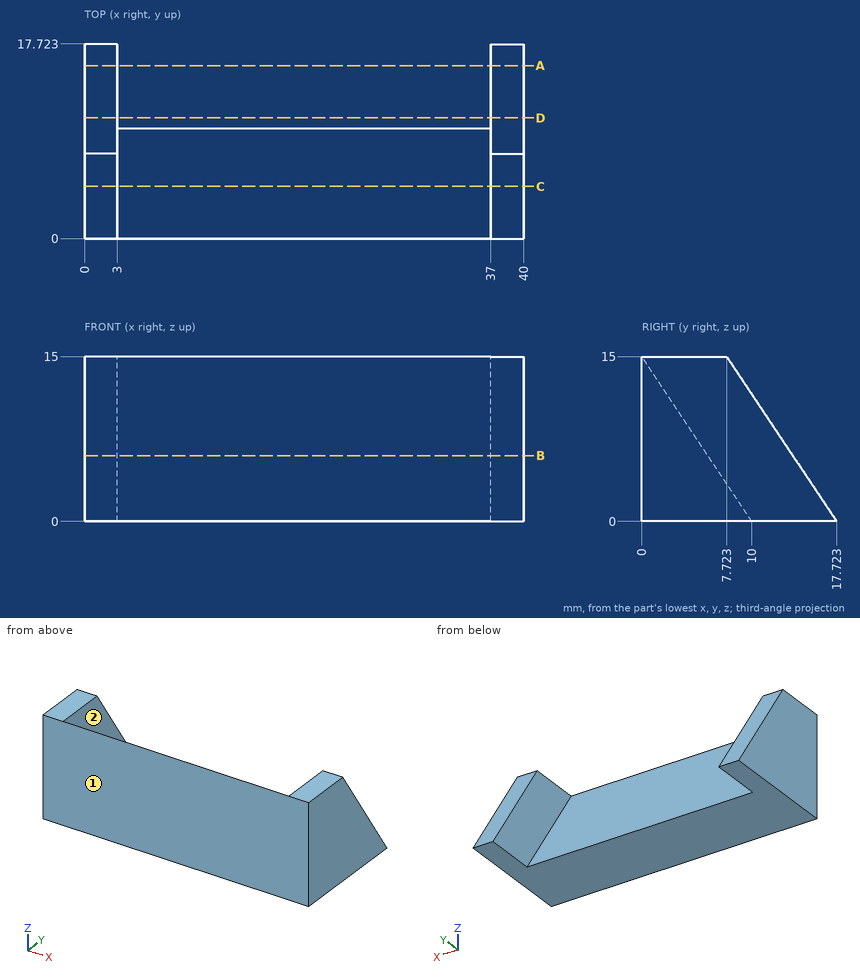
For this review, use the dimensioned drawing (mm, ordinates from the lowest corner) and the shaded views. A direction names the side the tool comes from. Coordinates: 2 decimals unless noted, no trailing zeros. Loops run counter-clockwise (first coordinate to the right, second up) from the corner with the lowest first, then second, coordinate; pieces in that order, holes last. Notation, with made-up numbers: (44.25, -34.5) -> (59.25, -34.5) arc R17 cw to (59.25, -14.5) -> close; hole circle Ø5 at (-37, -6). An arc over 180 degrees is marked (long way). Use a Markdown table: item, result. Add a question column.
1. Add section D-D on y = 11. Write out the cut boundary in (x, z).
2. Clearance check with flat-ended pins moving along their axes: pin 1 Ø8 at (y, z) = (13, 4.5) entering from -X; pin 2 Ø5 at (x, y) = (6, 9.5) entering from +Z; pin 3 Ø6 at (x, z) = (27.5, 6) entering from +Y; pin 4 Ø5 at (y, z) = (13.5, 13) entering from -X. State where each tip first meets the part, or that it passes through.
3. Add section B-B on z = 6. Write out the cut boundary in (x, y).
4. To check wall thickness, follow line 1 (X direction, y = 11, z = 3.5); line 2 (Z direction, x = 21.5, y = 8); line 3 (Z direction, x = 14, y = 3.25) (1 decimal). State the ranges of each line that lie inside material, in increasing order.
5. Machinability: for the marked faces 1 and 2, which of the approach directions +Z, -Z, +X, -X, +Y, -Y give a long, thin tool a straight path to every point of the face, cutting with its end or side? Answer none if there is none.
6. Add section C-C on y = 4.75. Write out the cut boundary in (x, z) (1 decimal), plus the area to 3 significant figures.
7. Add section A-A on y = 15.75. Write out the cut boundary in (x, z).
Returned:
| question | item | result |
|---|---|---|
| 1 | outline | (0, 0) -> (3, 0) -> (3, 10.08) -> (0, 10.08) -> close; (37, 0) -> (40, 0) -> (40, 10.08) -> (37, 10.08) -> close |
| 2 | pin 1 | stops at x = 0 |
| 2 | pin 2 | stops at z = 4.5 |
| 2 | pin 3 | stops at y = 8 |
| 2 | pin 4 | passes through |
| 3 | outline | (0, 0) -> (40, 0) -> (40, 13.72) -> (37, 13.72) -> (37, 6) -> (3, 6) -> (3, 13.72) -> (0, 13.72) -> close |
| 4 | line 1 | x = 0 to 3, 37 to 40 |
| 4 | line 2 | z = 0 to 3 |
| 4 | line 3 | z = 0 to 10.1 |
| 5 | face 1 | +Z, -Z, +X, -X, -Y |
| 5 | face 2 | +Z, +Y |
| 6 | outline | (0, 0) -> (40, 0) -> (40, 15) -> (37, 15) -> (37, 7.9) -> (3, 7.9) -> (3, 15) -> (0, 15) -> close |
| 6 | area | 358 mm² |
| 7 | outline | (0, 0) -> (3, 0) -> (3, 2.96) -> (0, 2.96) -> close; (37, 0) -> (40, 0) -> (40, 2.96) -> (37, 2.96) -> close |
